```python
from build123d import *

# Parameters (mm, degrees)
SKETCH1_R           = 38.1
BOSS_EXTRUDE1_DEPTH = 165.1
SKETCH2_R           = 3.9878
BOSS_EXTRUDE2_DEPTH = 25.4
FILLET1_R           = 3.81
SHELL2_OUTLINE_R    = 33.02
SHELL2_DEPTH        = 160.02


# Read off the part's stored shape, not the designer's step: Shell2
with BuildPart() as part:
    # Sketch1 → Boss-Extrude1 (new body)
    with BuildSketch(Plane(origin=(0, 0, 0), x_dir=(0, 0, -1), z_dir=(1, 0, 0))):
        Circle(SKETCH1_R)
    extrude(amount=BOSS_EXTRUDE1_DEPTH)

    # Sketch2 → Boss-Extrude2 (add)
    with BuildSketch(Plane(origin=(165.1, 0, 0), x_dir=(0, 0, -1), z_dir=(1, 0, 0))):
        Circle(SKETCH2_R)
    extrude(amount=BOSS_EXTRUDE2_DEPTH)

    # Fillet1
    fillet1_edges = [part.edges().sort_by_distance(p)[0] for p in [
        (0, 0, 38.1),
        (165.1, 0, 38.1),
    ]]
    fillet(fillet1_edges, radius=FILLET1_R)

    # Shell2 outline → Shell2 (cut)
    with BuildSketch(Plane.YZ):
        Circle(SHELL2_OUTLINE_R)
    extrude(amount=SHELL2_DEPTH, mode=Mode.SUBTRACT)


solid = part.part
```
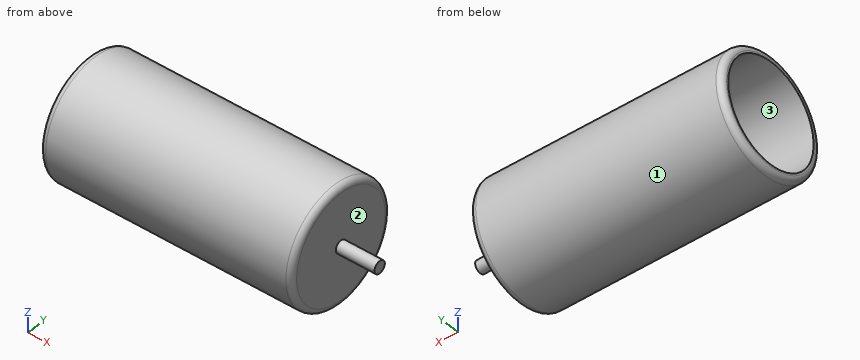
Design review of the part built by this model. Coordinates are the model's own, in mm. Face numbers are marked on the shaded views. Give positions to 0.01 mm unless a question says otherwise; leave off trailing zeros. Loops run counter-clockwise (first coordinate to the right, second up) from the corner with the lowest first, then second, coordinate; pieces in that order, holes last. Notation, with made-up numbers: M 8,16 L 15,16 A24 cw 15,26 Z; hole C 30.25,76.5 d3. An arc over 180 degrees is marked long. Return JSON: item names as keys, results as strings. Group by question number.
Item 1: For probe 1 along Y at (x, z) = (62, -1.5); probe 2 along X at (y, z) = (-33.5, 2); probe 3 along X at (y, z) = (-8, -4), list the stretches that pass through material, from the lowest coordinate up.
Item 2: We need section C-C (x = 79). Give the boundary of the cut face in (y, z).
Item 3: Mouldability with a two-part tool opening along Y and no side actions: class the marked faces 1, 2 and 3 as released by +Y, released by -Y, zero draft, split by the parting line, or undercut.
Item 4: We need section A-A (z = 0). Give the boundary of the cut face in (x, y), and give its area (3 significant figures).
Item 5: Insertion check: pin 1 Ø2 at (x, z) = (36, 19) entering from -Y; pin 2 Ø1 at (x, z) = (74, -9) entering from +Y; pin 3 Ø4 at (y, z) = (-16, 7.5) entering from -X. Each pin has a flat end and moves straight along its axis. Give the tip position at first contact, or say it passes through.
Output:
{
 "1": {"probe 1": "y = -38.07 to -32.99, 32.99 to 38.07", "probe 2": "x = 0 to 165.1", "probe 3": "x = 160.02 to 165.1"},
 "2": {"outline": "C 0,0 d76.2; hole C 0,0 d66.04"},
 "3": {"face 1": "split by the parting line", "face 2": "zero draft", "face 3": "undercut"},
 "4": {"outline": "M 0,-34.29 A3.81 ccw 3.81,-38.1 L 161.29,-38.1 A3.81 ccw 165.1,-34.29 L 165.1,-3.99 L 190.5,-3.99 L 190.5,3.99 L 165.1,3.99 L 165.1,34.29 A3.81 ccw 161.29,38.1 L 3.81,38.1 A3.81 ccw 0,34.29 L 0,33.02 L 160.02,33.02 L 160.02,-33.02 L 0,-33.02 Z", "area": "2,200 mm^2"},
 "5": {"pin 1": "stops at y = -33.58", "pin 2": "stops at y = 37.14", "pin 3": "stops at x = 160.02"}
}
